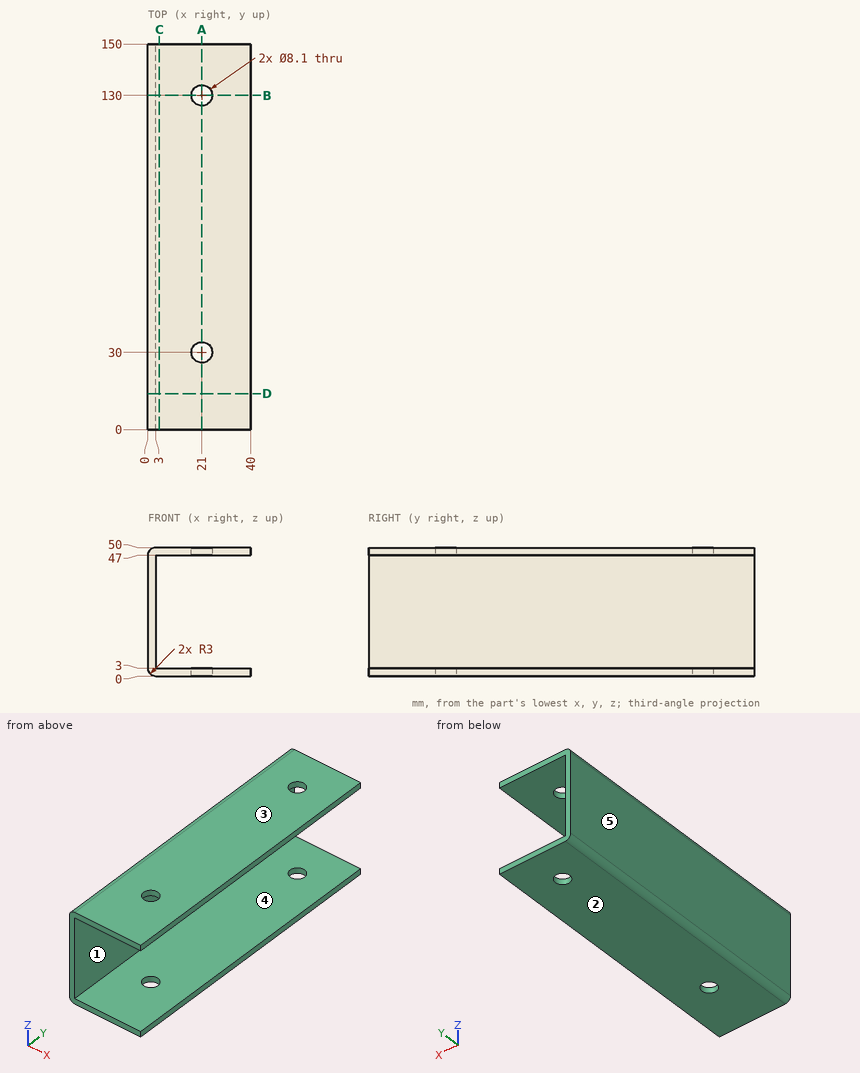
The figure shows three views and two pictorial views of one solid part (mm, origin at its lowest corner). Answer the questions. A direction names the side the tool comes from. Coordinates: 2 decimals unless noted, no trailing zeros. Loops run counter-clockwise (first coordinate to the right, second up) from the corner with the lowest first, then second, coordinate; pieces in that order, holes last.
1) Find section C-C on x = 4.5. Write down the section's boundary in (y, z).
2) Find section D-D on y = 14. Write down the section's boundary in (x, z), then the cut area to 3 significant figures.
3) A flat-ended cylindrical pin translates along its axis: pin 1 Ø13 at (y, z) = (52.5, 27.5) entering from +X. Find the tip coordinate at first contact, or state that the pin passes through.
4) Determine the mould class of the marked faces 3, 4 and 5 for opening direction Z: pulls with the +Z half, pulls with the -Z half, needs draft (parallel to the pull), parting line crosses it, or undercut.
5) Find the intervals of material crossed by L1, parallel to Y at x = 21, z = 1; L2, parallel to Z at x = 6, y = 134.5; L3, parallel to X at y = 81, z = 37, in increasing order.
6) Find section A-A on x = 21. Write down the section's boundary in (y, z).
7) A tool of negligible diameter and unlimited length cuts with its end or side. For the marked faces 1 and 2, from which of +Z, -Z, +X, -X, +Y, -Y can it reach the whole face along a straight path? Write none if from no direction.
8) Find section B-B on y = 130. Write down the section's boundary in (x, z).
Values:
1. outline: (0, 0) - (150, 0) - (150, 3) - (0, 3) - close; (0, 47) - (150, 47) - (150, 50) - (0, 50) - close
2. outline: (0, 3) arc R3 ccw to (3, 0) - (40, 0) - (40, 3) - (3, 3) - (3, 47) - (40, 47) - (40, 50) - (3, 50) arc R3 ccw to (0, 47) - close
2. area: 368 mm2
3. pin 1: stops at x = 3
4. face 3: pulls with the +Z half
4. face 4: undercut
4. face 5: needs draft
5. L1: y = 0 to 25.95, 34.05 to 125.95, 134.05 to 150
5. L2: z = 0 to 3, 47 to 50
5. L3: x = 0 to 3
6. outline: (0, 0) - (25.95, 0) - (25.95, 3) - (0, 3) - close; (0, 47) - (25.95, 47) - (25.95, 50) - (0, 50) - close; (34.05, 0) - (125.95, 0) - (125.95, 3) - (34.05, 3) - close; (34.05, 47) - (125.95, 47) - (125.95, 50) - (34.05, 50) - close; (134.05, 0) - (150, 0) - (150, 3) - (134.05, 3) - close; (134.05, 47) - (150, 47) - (150, 50) - (134.05, 50) - close
7. face 1: +X, +Y, -Y
7. face 2: -Z, +X, -X, +Y, -Y
8. outline: (0, 3) arc R3 ccw to (3, 0) - (16.95, 0) - (16.95, 3) - (3, 3) - (3, 47) - (16.95, 47) - (16.95, 50) - (3, 50) arc R3 ccw to (0, 47) - close; (25.05, 0) - (40, 0) - (40, 3) - (25.05, 3) - close; (25.05, 47) - (40, 47) - (40, 50) - (25.05, 50) - close
